For this review, take the finished solid that the model builds, in its own axes (mm). Give positions to 0.01 mm unless a question says otherwise; leave off trailing zeros. Loops run counter-clockwise (first coordinate to the right, second up) from the corner with the lowest first, then second, coordinate; pieces in that order, holes last. Notation, with made-up numbers: (53, 70) - (62, 70) arc R16 cw to (62, 85) - close; hole circle Ø4 at (-32.75, -21). An arc over 180 degrees is marked (long way). Answer in a Markdown table with one row per item.
```python
from build123d import *

# Parameters (mm, degrees)
MODEL_R             = 1.5
MODEL_R_2           = 2
MODEL_W             = 40
MODEL_H             = 40
MODEL_W_2           = 100
MODEL_H_2           = 15
EXTRUDE_1_DEPTH     = 3
SKETCH_2_W          = 96.919809602
SKETCH_2_H          = 88.226620572
EXTRUDE_2_DEPTH     = 3
SKETCH_3_W          = 55.118517674
SKETCH_3_H          = 61.40720761
EXTRUDE_3_DEPTH     = 3
SKETCH_4_R          = 3.5
CUT_EXTRUDE_4_DEPTH = 3
SKETCH_5_W          = 51.049365362
SKETCH_5_H          = 59.002708518
EXTRUDE_4_DEPTH     = 3


with BuildPart() as part:
    # Model → 凸台-拉伸1 (new body)
    with BuildSketch(Plane.XY):
        with BuildLine():
            Line((130, -77), (130, 77))
            ThreePointArc((130, 77), (129.121320344, 79.121320344), (127, 80))
            Line((127, 80), (-127, 80))
            ThreePointArc((-127, 80), (-129.121320344, 79.121320344), (-130, 77))
            Line((-130, 77), (-130, -77))
            ThreePointArc((-130, -77), (-129.121320344, -79.121320344), (-127, -80))
            Line((-127, -80), (127, -80))
            ThreePointArc((127, -80), (129.121320344, -79.121320344), (130, -77))
        make_face()
        with Locations((0, 40.4)):
            Circle(MODEL_R, mode=Mode.SUBTRACT)
        with Locations((40.4, 0)):
            Circle(MODEL_R, mode=Mode.SUBTRACT)
        with Locations((0, -40.4)):
            Circle(MODEL_R, mode=Mode.SUBTRACT)
        with Locations((-40.4, 0)):
            Circle(MODEL_R, mode=Mode.SUBTRACT)
        with Locations((-110, 73)):
            Circle(MODEL_R_2, mode=Mode.SUBTRACT)
        with Locations((110, 73)):
            Circle(MODEL_R_2, mode=Mode.SUBTRACT)
        with Locations((110, -73)):
            Circle(MODEL_R_2, mode=Mode.SUBTRACT)
        with Locations((-110, -73)):
            Circle(MODEL_R_2, mode=Mode.SUBTRACT)
        with Locations((-120, 73)):
            Circle(MODEL_R_2, mode=Mode.SUBTRACT)
        with Locations((120, 73)):
            Circle(MODEL_R_2, mode=Mode.SUBTRACT)
        with Locations((-120, -73)):
            Circle(MODEL_R_2, mode=Mode.SUBTRACT)
        with Locations((120, -73)):
            Circle(MODEL_R_2, mode=Mode.SUBTRACT)
        with Locations((-100, 73)):
            Circle(MODEL_R_2, mode=Mode.SUBTRACT)
        with Locations((100, 73)):
            Circle(MODEL_R_2, mode=Mode.SUBTRACT)
        with Locations((100, -73)):
            Circle(MODEL_R_2, mode=Mode.SUBTRACT)
        with Locations((-100, -73)):
            Circle(MODEL_R_2, mode=Mode.SUBTRACT)
        with Locations((-90, 0)):
            Rectangle(MODEL_W, MODEL_H, mode=Mode.SUBTRACT)
        with Locations((90, 0)):
            Rectangle(MODEL_W, MODEL_H, mode=Mode.SUBTRACT)
        with Locations((0, 60)):
            Rectangle(MODEL_W_2, MODEL_H_2, mode=Mode.SUBTRACT)
        with Locations((0, -60)):
            Rectangle(MODEL_W_2, MODEL_H_2, mode=Mode.SUBTRACT)
        with BuildLine():
            Line((28.543233286, -28.543233286), (28.543233286, -23.543233286))
            ThreePointArc((28.543233286, -23.543233286), (-26.162950904, 26.162950904), (23.543233286, -28.543233286))
            Line((23.543233286, -28.543233286), (28.543233286, -28.543233286))
        make_face(mode=Mode.SUBTRACT)
    extrude(amount=EXTRUDE_1_DEPTH)

    # 草图2 → 凸台-拉伸2 (add)
    with BuildSketch(Plane.XY.offset(3)):
        Rectangle(SKETCH_2_W, SKETCH_2_H)
    extrude(amount=-EXTRUDE_2_DEPTH)

    # 草图3 → 凸台-拉伸3 (add)
    with BuildSketch(Plane.XY.offset(3)):
        with Locations((88.781504979, -1.572172484)):
            Rectangle(SKETCH_3_W, SKETCH_3_H)
    extrude(amount=-EXTRUDE_3_DEPTH)

    # 草图4 → 切除-拉伸4 (cut)
    with BuildSketch(Plane.XY.offset(3)):
        with Locations((100, 0)):
            Circle(SKETCH_4_R)
    extrude(amount=-CUT_EXTRUDE_4_DEPTH, mode=Mode.SUBTRACT)

    # 草图5 → 凸台-拉伸4 (add)
    with BuildSketch(Plane.XY.offset(3)):
        with Locations((-90.446158197, 0)):
            Rectangle(SKETCH_5_W, SKETCH_5_H)
    extrude(amount=-EXTRUDE_4_DEPTH)


solid = part.part
```
1. We need section B-B, the plane x = 25. Give the boundary of the cut face in (y, z), and give its area (3 significant figures).
Values:
| item | result |
|---|---|
| outline | (-80, 0) - (-67.5, 0) - (-67.5, 3) - (-80, 3) - close; (-52.5, 0) - (52.5, 0) - (52.5, 3) - (-52.5, 3) - close; (67.5, 0) - (80, 0) - (80, 3) - (67.5, 3) - close |
| area | 390 mm^2 |
2. Mouldability with a two-part tool opening along X and no side actions: class faces 1 (the face through (103.233, -1.341, 1.521)), 2 (the face through (-2, 1, 0)) as released by +X, released by -X, zero draft, split by the parting line, or undercut.
Values:
| item | result |
|---|---|
| face 1 | undercut |
| face 2 | zero draft |
3. We need section C-C, the plane z = 0.7. Count the separate pieces of the cut face and the enclosed holes in it, and give its area (3 significant figures).
Values:
| item | result |
|---|---|
| separate pieces | 1 |
| enclosed holes | 15 |
| area | 38,400 mm^2 |
4. We need section D-D, the plane y = 0. Give the boundary of the cut face in (x, z).
Values:
| item | result |
|---|---|
| outline | (-130, 0) - (96.5, 0) - (96.5, 3) - (-130, 3) - close; (103.5, 0) - (130, 0) - (130, 3) - (103.5, 3) - close |
5. Clearance check with a flat-ended pin moving along its axis: pin 1 (10 mm diameter, centred on x = -42.5, y = -41.5, fed in from -Z). State where the tip first meets the part, or that it passes through.
Values:
| item | result |
|---|---|
| pin 1 | stops at z = 0 |
6. Wall thickness on line 1 (Y direction, x = 20, z = 1.6); line 2 (Y direction, x = 120, z = 1.3); line 3 (X direction, y = 66, z = 1.2): over which ranges is each line inside the solid? List them lowest first. Write a range as [from, to].
Values:
| item | result |
|---|---|
| line 1 | y = [-80, -67.5], [-52.5, 52.5], [67.5, 80] |
| line 2 | y = [-80, -75], [-71, 71], [75, 80] |
| line 3 | x = [-130, -50], [50, 130] |
7. We need section A-A, the plane y = -62. Give the boundary of the cut face in (x, z).
Values:
| item | result |
|---|---|
| outline | (-130, 0) - (-50, 0) - (-50, 3) - (-130, 3) - close; (50, 0) - (130, 0) - (130, 3) - (50, 3) - close |
